CAD build for the part. Positions are in the model's coordinates, mm. A direction names the side the tool comes from. Coordinates: 2 decimals unless noted, no trailing zeros. Write each loop counter-clockwise with the first axis right and the second up, starting at its lowest first coordinate (ties: lowest second). Pieces come first, ordered by that corner, then holes. Notation, with made-up numbers: (23.5, 3) -> (80.5, 3) arc R23 ccw to (80.5, 27) -> close; hole circle Ø10 at (14.25, 84.5). An arc over 180 degrees is marked (long way). Answer as CSV lines item,"result". Start each with the question number.
```python
from build123d import *

# Parameters (mm, degrees)
BOSS_EXTRUDE1_DEPTH = 76.2
SKETCH2_R           = 6.35
CUT_EXTRUDE1_DEPTH  = 83.55
SKETCH3_W           = 25.4
SKETCH3_H           = 63.5
CUT_EXTRUDE2_DEPTH  = 45.4500001


with BuildPart() as part:
    # Sketch1 → Boss-Extrude1 (new body)
    with BuildSketch(Plane(origin=(0, 0, 0), x_dir=(1, 0, 0), z_dir=(0, 1, 0))):
        with BuildLine():
            Line((0, 82.55), (0, 44.45))
            ThreePointArc((0, 44.45), (44.45, 0), (0, -44.45))
            Line((0, -44.45), (0, -82.55))
            ThreePointArc((0, -82.55), (82.55, 0), (0, 82.55))
        make_face()
    extrude(amount=BOSS_EXTRUDE1_DEPTH)

    # Sketch2 → Cut-Extrude1 (cut, through all)
    with BuildSketch(Plane.ZY):
        with Locations((-63.5, 57.15)):
            Circle(SKETCH2_R)
        with Locations((-63.5, 19.05)):
            Circle(SKETCH2_R)
        with Locations((63.5, 19.05)):
            Circle(SKETCH2_R)
        with Locations((63.5, 57.15)):
            Circle(SKETCH2_R)
    extrude(amount=-CUT_EXTRUDE1_DEPTH, mode=Mode.SUBTRACT)

    # Sketch3 → Cut-Extrude2 (cut, through all)
    with BuildSketch(Plane.ZY.offset(-38.1)):
        with Locations((63.5, 38.1)):
            Rectangle(SKETCH3_W, SKETCH3_H)
        with Locations((-63.5, 38.1)):
            Rectangle(SKETCH3_W, SKETCH3_H)
    extrude(amount=-CUT_EXTRUDE2_DEPTH, mode=Mode.SUBTRACT)


solid = part.part
```
1. Cut at B-B (y = 19.05). Give the cut face in (x, z).
2. Mould opens along Y. For faces 4 (the face through (50, 76.2, -1)), 5 (the face through (0, 38, 63)), 6 (the face through (18.78, 23.34, -68.18)) say: pulls with the +Y half, pulls with the -Y half, needs draft (parallel to the pull), parting line crosses it, or undercut.
3. Wall check: line 1 (Y direction, x = 17.5, z = -63.5); line 2 (X direction, y = 52.5, z = -70); line 3 (Z direction, x = 14.5, y = 30). Give the ranges that are in metal, low to high.
4. Flat gauge pins, fed straight in: P1, Ø16.5, axis at y = 19.05, z = -63.5, coming from the +X side; P2, Ø5, axis at y = 41.5, z = 22.5, coming from the -X side; P3, Ø5, axis at x = 47.5, y = 43.5, coming from the -Z side; P4, Ø11, axis at x = 49.5, z = 57, coming from the -Y side. Where does each tip first touch, or does it go through?
5. Cut at A-A (x = 26.5). Give the cut face in (y, z).
6. Cut at D-D (z = -63.5). Give the cut face in (x, y), then the cut area to 3 significant figures.
7. Cut at C-C (y = 47.5). Give the cut face in (x, z).
8. Tool access for faces 1 (the face through (82.53, 37.57, 1.82)), 2 (the face through (51, 38, -50.8)), 3 (the face through (48, 6.35, 59)): list every direction of +Z, -Z, +X, -X, +Y, -Y with a clear straight run to the whole face (end or side of a thin tool).
Geometry check:
1,outline,"(0, -82.55) arc R82.55 ccw to (38.1, -73.23) -> (38.1, -69.85) -> (0, -69.85) -> close; (0, -57.15) -> (38.1, -57.15) -> (38.1, -50.8) -> (65.07, -50.8) arc R82.55 ccw to (65.07, 50.8) -> (38.1, 50.8) -> (38.1, 57.15) -> (0, 57.15) -> (0, 44.45) arc R44.45 cw to (0, -44.45) -> close; (0, 69.85) -> (38.1, 69.85) -> (38.1, 73.23) arc R82.55 ccw to (0, 82.55) -> close"
2,face 4,"pulls with the +Y half"
2,face 5,"needs draft"
2,face 6,"undercut"
3,line 1,"0 to 12.7, 25.4 to 50.8, 63.5 to 76.2"
3,line 2,"0 to 38.1"
3,line 3,"-81.27 to -42.02, 42.02 to 81.27"
4,P1,"x = 38.1"
4,P2,"x = 36.75"
4,P3,"z = -50.8"
4,P4,"y = 0"
5,outline,"(0, -78.18) -> (76.2, -78.18) -> (76.2, -35.69) -> (0, -35.69) -> close; (0, 35.69) -> (76.2, 35.69) -> (76.2, 78.18) -> (0, 78.18) -> close; hole circle Ø12.7 at (19.05, -63.5); hole circle Ø12.7 at (19.05, 63.5); hole circle Ø12.7 at (57.15, -63.5); hole circle Ø12.7 at (57.15, 63.5)"
6,outline,"(0, 0) -> (52.75, 0) -> (52.75, 6.35) -> (38.1, 6.35) -> (38.1, 12.7) -> (0, 12.7) -> close; (0, 25.4) -> (38.1, 25.4) -> (38.1, 50.8) -> (0, 50.8) -> close; (0, 63.5) -> (38.1, 63.5) -> (38.1, 69.85) -> (52.75, 69.85) -> (52.75, 76.2) -> (0, 76.2) -> close"
6,area,"2,120 mm²"
7,outline,"(0, -82.55) arc R82.55 ccw to (38.1, -73.23) -> (38.1, -50.8) -> (65.07, -50.8) arc R82.55 ccw to (65.07, 50.8) -> (38.1, 50.8) -> (38.1, 73.23) arc R82.55 ccw to (0, 82.55) -> (0, 44.45) arc R44.45 cw to (0, -44.45) -> close"
8,face 1,"+X, +Y, -Y"
8,face 2,"-Z, +X"
8,face 3,"+Z, +X"
